```python
from build123d import *

# Parameters (mm, degrees)
SKETCH_2_R          = 94
EXTRUDE_1_DEPTH     = 5
SKETCH_3_W          = 204.518128244
SKETCH_3_H          = 25
CUT_EXTRUDE_1_DEPTH = 134.311664906
SKETCH_4_R          = 11
CUT_EXTRUDE_2_DEPTH = 134.311664906
SKETCH_5_R          = 60
CUT_EXTRUDE_3_DEPTH = 2
M8X1_25_1_D         = 6.8
M8X1_25_1_DEPTH     = 19.75
M8X1_25_1_TIP       = 2.042926105
SKETCH_8_R          = 4.5
CUT_EXTRUDE_4_DEPTH = 134.311664906
CHAMFER_1_SIZE      = 2


with BuildPart() as part:
    # 草图2 → 凸台-拉伸1 (new, symmetric)
    with BuildSketch(Plane(origin=(0, 0, 0), x_dir=(1, 0, 0), z_dir=(0, 1, 0))):
        with Locations(Location((0, 0, 0), (0, 0, 270))):
            Circle(SKETCH_2_R)
    extrude(amount=EXTRUDE_1_DEPTH, both=True)

    # 草图3 → 切除-拉伸1 (cut, through all)
    with BuildSketch(Plane(origin=(0, 5, 0), x_dir=(1, 0, 0), z_dir=(0, 1, 0))):
        with Locations((5.966826679, 81.5)):
            Rectangle(SKETCH_3_W, SKETCH_3_H)
    extrude(amount=-CUT_EXTRUDE_1_DEPTH, mode=Mode.SUBTRACT)

    # 草图4 → 切除-拉伸2 (cut, through all)
    with BuildSketch(Plane(origin=(0, 5, 0), x_dir=(1, 0, 0), z_dir=(0, 1, 0))):
        with Locations(Location((0, 0, 0), (0, 0, 270))):
            Circle(SKETCH_4_R)
    extrude(amount=-CUT_EXTRUDE_2_DEPTH, mode=Mode.SUBTRACT)

    # 草图5 → 切除-拉伸3 (cut)
    with BuildSketch(Plane(origin=(0, 5, 0), x_dir=(1, 0, 0), z_dir=(0, 1, 0))):
        with Locations(Location((0, 0, 0), (0, 0, 270))):
            Circle(SKETCH_5_R)
    cut_extrude_3 = extrude(amount=-CUT_EXTRUDE_3_DEPTH, mode=Mode.SUBTRACT)

    # 镜向1: 切除-拉伸3 across plane
    add(cut_extrude_3.mirror(Plane.ZX), mode=Mode.SUBTRACT)

    # M8x1.25 螺纹孔1
    with Locations(Plane(origin=(0, 5, 0), x_dir=(-1, 0, 0), z_dir=(0, 1, 0))):
        with Locations((72, -38.5), (-72, -38.5), (72, 38.5), (-72, 38.5)):
            Hole(M8X1_25_1_D / 2, depth=M8X1_25_1_DEPTH)
            with Locations((0, 0, -(M8X1_25_1_DEPTH + M8X1_25_1_TIP / 2))):  # 118° drill point
                Cone(0, M8X1_25_1_D / 2, M8X1_25_1_TIP, mode=Mode.SUBTRACT)

    # 草图8 → 切除-拉伸4 (cut, through all)
    with BuildSketch(Plane(origin=(0, 5, 0), x_dir=(1, 0, 0), z_dir=(0, 1, 0))):
        with Locations(Location((0, -85, 0), (0, 0, 270))):
            Circle(SKETCH_8_R)
    extrude(amount=-CUT_EXTRUDE_4_DEPTH, mode=Mode.SUBTRACT)

    # 倒角1
    chamfer_1_edges = [part.edges().sort_by_distance(p)[0] for p in [
        (0, 5, -60),
        (0, 3, -11),
        (0, -5, -60),
        (0, -3, -11),
        (0, -5, 94),
        (0, 5, 94),
    ]]
    chamfer(chamfer_1_edges, length=CHAMFER_1_SIZE - 0.0001)  # a hair under: the kernel refuses the full size


solid = part.part
```
Verification items for the finished model (mm, model axes). A direction names the side the tool comes from. Round coordinates to 2 decimals unless told otherwise and drop trailing zeros.
1) Depth check by flat-ended pin: pin 1 (3 mm diameter, centred on x = 14.5, z = 23.5, fed in from -Y); pin 2 (1 mm diameter, centred on x = -34.5, z = 41.5, fed in from +Y); pin 3 (6 mm diameter, centred on x = -72, z = -38.5, fed in from +Y); pin 4 (1.5 mm diameter, centred on x = 15, y = 4, fed in from +Z). Enter the tip coordinate at first touch or a pass-through.
Geometry says:
pin 1: stops at y = -3
pin 2: stops at y = 3
pin 3: passes through
pin 4: stops at z = 92.55
2) Cross-section at A-A, the plane x = 0. Give the number of separate pieces and of enclosed holes in the cut face, plus the area to 3 significant figures.
Geometry says:
separate pieces: 3
enclosed holes: 0
area: 908 mm2
3) Draft check along Z on faces 4 (the flat face through (42, -5, 46)), 5 (the flat face through (-1, 0, -69)), 6 (the conical face through (3.126, 4.681, 92.266)), 7 (the cylindrical face through (-74.506, -0.07, 40.798)). Enter one of: +Z half, -Z half, draft (parallel to the pull), parting line (faces both ways), or undercut.
Geometry says:
face 4: draft
face 5: -Z half
face 6: parting line
face 7: undercut
4) Tool access check on faces 1 (the flat face through (14, -3, -1)), 2 (the cylindrical face through (-72.44, -0.07, -35.13)), 3 (the flat face through (14, 3, -1)). Record the directions out of +Z, -Z, +X, -X, +Y, -Y that give a thin tool (end or side, any length) a straight path to the whole face; none if there is none.
Geometry says:
face 1: -Y
face 2: +Y, -Y
face 3: +Y
5) Material ranges on line 1 (Z direction, x = 72, y = -2.5); line 2 (Y direction, x = 43, z = -26); line 3 (X direction, y = -0.3, z = 0), recorded low to high.
Geometry says:
line 1: z = -60.43 to -41.9, -35.1 to 35.1, 41.9 to 60.43
line 2: y = -3 to 3
line 3: x = -94 to -11, 11 to 94
